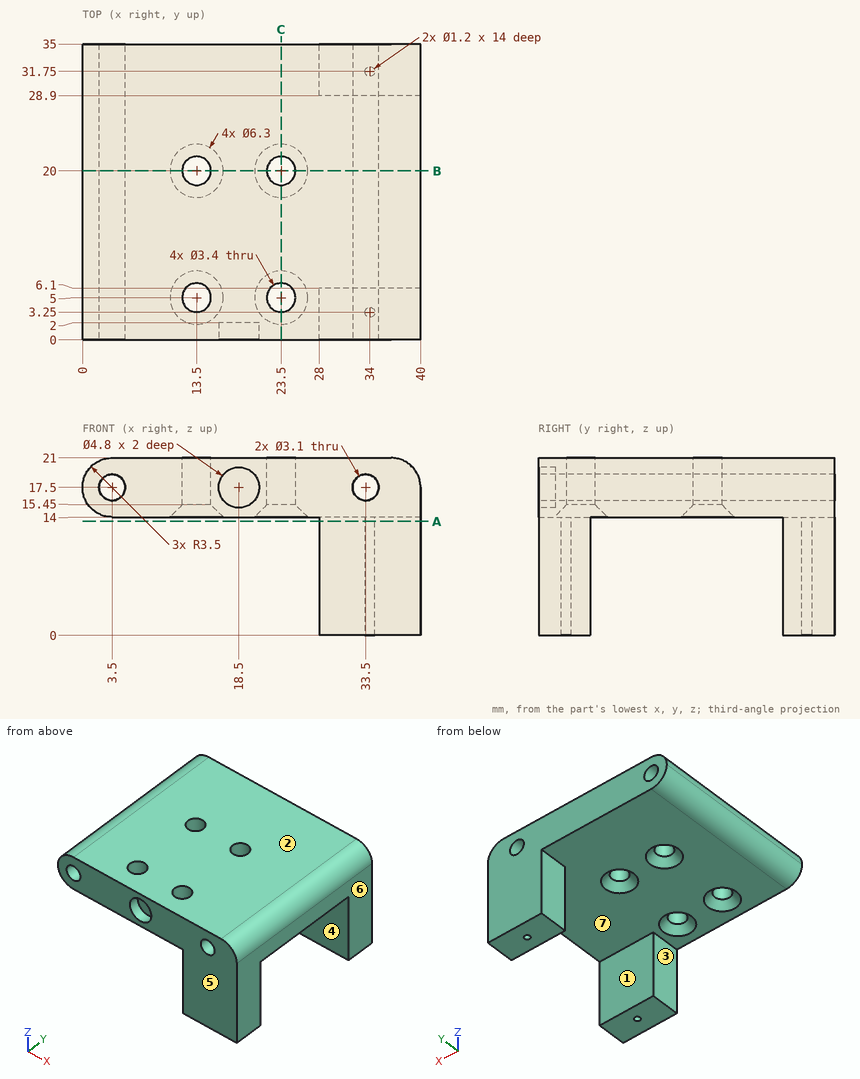
Geometry: see drawing. Coordinates: mm, zero at the bounding-box minimum. A direction names the side the tool comes from. Give positions to 0.01 mm unless a question says otherwise; leave off trailing zeros. Loops run counter-clockwise (first coordinate to the right, second up) from the corner with the lowest first, then second, coordinate; pieces in that order, holes last. Notation, with made-up numbers: (74.5, 84.25) - (93.5, 84.25) arc R28 cw to (93.5, 105.25) - close; hole circle Ø11 at (-37.5, 12.25). An arc over 180 degrees is marked (long way). Use CSV: the item, a comma, the result in double quotes.
1) Cut plane A-A (z = 13.5). Output: boundary loops of the cut face in (x, y).
Worked out:
outline,"(28, 0) - (40, 0) - (40, 6.1) - (28, 6.1) - close; (28, 28.9) - (40, 28.9) - (40, 35) - (28, 35) - close; hole circle Ø1.2 at (34, 3.25); hole circle Ø1.2 at (34, 31.75)"
2) Set-up query: the marked faces 1, 2 and 3. Return all of +Z, -Z, +X, -X, +Y, -Y with unobstructed straight access to the full face (end or side cutting, diameter ignored); none if empty.
Worked out:
face 1,"-Z, +X, -X"
face 2,"+Z, +X, -X, +Y, -Y"
face 3,"-Z, -X, +Y, -Y"
3) Pin query (flat end, axial travel): P1, Ø4.5, axis at x = 13.5, y = 5, coming from the -Z side; P2, Ø5, axis at y = 3, z = 5, coming from the -X side; P3, Ø1.1, axis at x = 34, y = 3.25, coming from the -Z side. Return the tip coordinate at first contact, or that it passes through.
Worked out:
P1,"stops at z = 14.9"
P2,"stops at x = 28"
P3,"stops at z = 14"
4) Cut plane C-C (x = 23.5). Output: boundary loops of the cut face in (y, z).
Worked out:
outline,"(0, 14) - (1.85, 14) - (3.3, 15.45) - (3.3, 21) - (0, 21) - close; (6.7, 15.45) - (8.15, 14) - (16.85, 14) - (18.3, 15.45) - (18.3, 21) - (6.7, 21) - close; (21.7, 15.45) - (23.15, 14) - (35, 14) - (35, 21) - (21.7, 21) - close"
5) Line query: line 1 (X direction, y = 1.6, z = 17.5); line 2 (Y direction, x = 13.5, z = 17.6); line 3 (Y direction, x = 34, z = 10.25). Output: solid intervals per line, ascending.
Worked out:
line 1,"x = 0 to 1.95, 5.05 to 16.1, 20.9 to 31.95, 35.05 to 40"
line 2,"y = 0 to 3.3, 6.7 to 18.3, 21.7 to 35"
line 3,"y = 0 to 2.65, 3.85 to 6.1, 28.9 to 31.15, 32.35 to 35"
6) Mould query, pull axis Y, two halves, no side actions, for the marked faces 4, 5, 6 and 7. Classes: +Y half, -Y half, draft (parallel to the pull), parting line (faces both ways), or undercut.
Worked out:
face 4,"undercut"
face 5,"-Y half"
face 6,"draft"
face 7,"undercut"
7) Cut plane B-B (y = 20). Count the separate pieces of the cut face and the enclosed holes in it, and give its area (3 significant figures).
Worked out:
separate pieces,"3"
enclosed holes,"2"
area,"205 mm^2"
